Part print with two shaded views. Sizes in mm from the minimum x, y, z corner. Coordinates: 2 decimals unless noted, no trailing zeros. Loops run counter-clockwise (first coordinate to the right, second up) from the corner with the lowest first, then second, coordinate; pieces in that order, holes last.
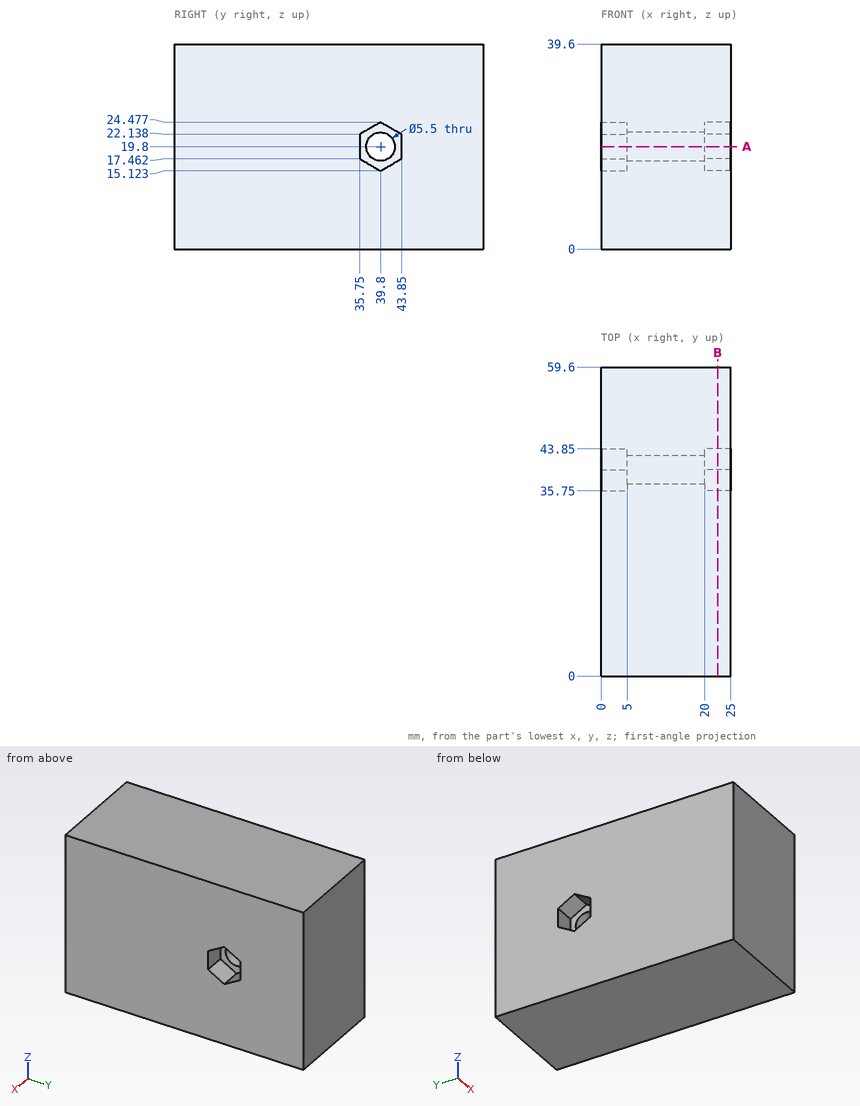
Q1. Drill centre lines: line 1 (Y direction, x = 13.25, z = 19.8); line 2 (Z direction, x = 16.75, y = 39.8); line 3 (Z direction, x = 18, y = 42). Where is each one in solid material? Low to high.
Answers:
line 1: y = 0 to 37.05, 42.55 to 59.6
line 2: z = 0 to 17.05, 22.55 to 39.6
line 3: z = 0 to 18.15, 21.45 to 39.6
Q2. Slice it at A-A (z = 19.8). List the corners of the cut face in (x, y).
Answers:
outline: (0, 0) - (25, 0) - (25, 35.75) - (20, 35.75) - (20, 37.05) - (5, 37.05) - (5, 35.75) - (0, 35.75) - close; (0, 43.85) - (5, 43.85) - (5, 42.55) - (20, 42.55) - (20, 43.85) - (25, 43.85) - (25, 59.6) - (0, 59.6) - close
Q3. Slice it at B-B (x = 22.5). List the corners of the cut face in (y, z), and give its area (3 significant figures).
Answers:
outline: (0, 0) - (59.6, 0) - (59.6, 39.6) - (0, 39.6) - close; hole (35.75, 17.46) - (39.8, 15.12) - (43.85, 17.46) - (43.85, 22.14) - (39.8, 24.48) - (35.75, 22.14) - close
area: 2,300 mm2
